Model file for the job. Use its own axes, mm. A direction names the side the tool comes from. Round coordinates to 2 decimals unless told otherwise and drop trailing zeros. Loops run counter-clockwise (first coordinate to the right, second up) from the corner with the lowest first, then second, coordinate; pieces in that order, holes last. Notation, with made-up numbers: M 66,17.5 L 86,17.5 A11 ccw 86,38.5 Z; hole C 76,87.25 d7. An arc over 180 degrees is marked long. Use a Markdown table: item, result. Add a question column.
Q1. Probe line 1 (X direction, y = 24, z = -9); line 2 (X direction, y = 4, z = 0); line 3 (Y direction, x = -8.4, z = 0). List the from-to ranges inside material, lowest first. Write a range as from..to.
Q2. Tool access for faces 5 (the face through (1.3, 3.45, -4.1)), 6 (the face through (-13, 6.9, 0)), 7 (the face through (11.13, 18.678, 0.423)), 8 (the face through (1, 3, -15)), 9 (the face through (10.8, 18, 0)): list every direction of +Z, -Z, +X, -X, +Y, -Y with a clear straight run to the whole face (end or side of a thin tool).
Q3. Mould opens along X. For faces 1 (the face through (11.62, 25.24, 0.74)), 2 (the face through (-10.8, 18, 0)), 3 (the face through (12.52, 15.3, -13.99)), 4 (the face through (-1.88, 5.2, 5.96)) say: +X half, -X half, draft (parallel to the pull), parting line (faces both ways), or undercut.
Q4. Cut at A-A (x = 0). Give the cut face in (y, z).
Q5. Cut at C-C (y = 13). Give the cut face in (x, z), plus the area to 3 significant figures.
Q6. Cut at D-D (y = 21.9). Give the cut face in (x, z), plus the area to 3 significant figures.
Q7. Pin check, flat tips, straight feed: pin 1 (6 mm diameter, centred on y = 21.9, z = 0, fed in from -X); pin 2 (10 mm diameter, centred on x = -4.5, y = 20.5, fed in from +Z); pin 3 (8.5 mm diameter, centred on y = 21.9, z = 0, fed in from +X); pin 4 (6.5 mm diameter, centred on x = 0, z = 0, fed in from +Y). Stop position of each tip, or through.
Q8. Cut at B-B (z = 0). Give the cut face in (x, y), plus the area to 3 significant figures.
from build123d import *

# Parameters (mm, degrees)
SKETCH_1_W               = 28.4
SKETCH_1_H               = 30
EXTRUDE_1_DEPTH          = 6.9
EXTRUDE_2_DEPTH          = 25
SKETCH_4_W               = 18.2
SKETCH_4_H               = 28.1
CUT_EXTRUDE_1_DEPTH      = 16
CUT_EXTRUDE_1_DEPTH_BACK = 16
CHAMFER_1_SIZE           = 2
HOLE_WIZARD_M61_D        = 5
HOLE_WIZARD_M61_DEPTH    = 3.4


with BuildPart() as part:
    # Эскиз1 → Бобышка-Вытянуть1 (new body)
    with BuildSketch(Plane(origin=(0, 0, 0), x_dir=(1, 0, 0), z_dir=(0, 1, 0))):
        Rectangle(SKETCH_1_W, SKETCH_1_H)
    extrude(amount=EXTRUDE_1_DEPTH)

    # Эскиз2 → Вырез-Повернуть1 (revolve, cut)
    with BuildSketch(Plane.XY, mode=Mode.PRIVATE) as cut_revolve_1_sk:
        Polygon((-4, 0), (-4, 3.45), (-6.25, 3.45), (-6.25, 6.9), (0, 6.9), (0, 0), align=None)
    revolve(cut_revolve_1_sk.sketch.rotate(Axis((0, 6.9, 0), (0, -1, 0)), 270), axis=Axis((0, 6.9, 0), (0, -1, 0)), mode=Mode.SUBTRACT)  # turned: the seam where the file's is

    # Эскиз3 → Бобышка-Вытянуть2 (add)
    with BuildSketch(Plane(origin=(14.2, 0, 0), x_dir=(0, 0, -1), z_dir=(1, 0, 0))):
        with BuildLine():
            Line((-15, 6.9), (-13.006126808, 23.465460141))
            ThreePointArc((-13.006126808, 23.465460141), (0, 35), (13.006126808, 23.465460141))
            Line((13.006126808, 23.465460141), (15, 6.9))
            Line((15, 6.9), (-15, 6.9))
        make_face()
    extrude(amount=-EXTRUDE_2_DEPTH)

    # Эскиз4 → Вырез-Вытянуть1 (cut, two sides)
    with BuildSketch(Plane.XY) as cut_extrude_1_sk:
        with Locations((1.7, 20.95)):
            Rectangle(SKETCH_4_W, SKETCH_4_H)
    extrude(amount=CUT_EXTRUDE_1_DEPTH, mode=Mode.SUBTRACT)
    extrude(cut_extrude_1_sk.sketch, amount=-CUT_EXTRUDE_1_DEPTH_BACK, mode=Mode.SUBTRACT)

    # Фаска1
    chamfer_1_edges = [part.edges().sort_by_distance(p)[0] for p in [
        (-14.2, 3.45, -15),
        (-14.2, 3.45, 15),
    ]]
    chamfer(chamfer_1_edges, length=CHAMFER_1_SIZE)

    # Отверстие обработанное метчиком M61
    with Locations(Plane.ZY.offset(10.8)):
        with Locations((0, 21.9)):
            Hole(HOLE_WIZARD_M61_D / 2, depth=HOLE_WIZARD_M61_DEPTH)

    # Эскиз10 → Зенковка для винта с полупотайной головкой 1 (revolve, cut)
    with BuildSketch(Plane(origin=(14.2, 21.9, 0), x_dir=(0, 0, -1), z_dir=(0, 1, 0))):
        Polygon((0, 0), (0, 3.4), (3.25, 3.4), (3.25, 2.75), (6, 0), align=None)
    revolve(axis=Axis((20.55, 21.9, 0), (-1, 0, 0)), mode=Mode.SUBTRACT)


solid = part.part
Checked values:
| question | item | result |
|---|---|---|
| 1 | line 1 | x = -10.8..-7.4, 10.8..14.2 |
| 1 | line 2 | x = -14.2..-6.25, 6.25..14.2 |
| 1 | line 3 | y = 0..19.4, 24.4..35 |
| 2 | face 5 | +Y |
| 2 | face 6 | +Z, -Z, -X, +Y |
| 2 | face 7 | +X |
| 2 | face 8 | -Z, +X, -X, +Y, -Y |
| 2 | face 9 | +Z, -Z, +Y |
| 3 | face 1 | +X half |
| 3 | face 2 | -X half |
| 3 | face 3 | draft |
| 3 | face 4 | undercut |
| 4 | outline | M 0,-15 L 6.9,-15 L 6.9,-6.25 L 3.45,-6.25 L 3.45,-4 L 0,-4 Z; M 0,4 L 3.45,4 L 3.45,6.25 L 6.9,6.25 L 6.9,15 L 0,15 Z |
| 5 | outline | M -10.8,-14.27 L -7.4,-14.27 L -7.4,14.27 L -10.8,14.27 Z; M 10.8,-14.27 L 14.2,-14.27 L 14.2,14.27 L 10.8,14.27 Z |
| 5 | area | 194 mm^2 |
| 6 | outline | M -10.8,-13.19 L -7.4,-13.19 L -7.4,-2.5 L -10.8,-2.5 Z; M -10.8,2.5 L -7.4,2.5 L -7.4,13.19 L -10.8,13.19 Z; M 10.8,-13.19 L 14.2,-13.19 L 14.2,-6 L 11.45,-3.25 L 10.8,-3.25 Z; M 10.8,3.25 L 11.45,3.25 L 14.2,6 L 14.2,13.19 L 10.8,13.19 Z |
| 6 | area | 133 mm^2 |
| 7 | pin 1 | stops at x = -10.8 |
| 7 | pin 2 | stops at z = 13.85 |
| 7 | pin 3 | stops at x = 12.45 |
| 7 | pin 4 | passes through |
| 8 | outline | M -14.2,0 L -4,0 L -4,3.45 L -6.25,3.45 L -6.25,6.9 L -7.4,6.9 L -7.4,19.4 L -10.8,19.4 L -10.8,6.9 L -14.2,6.9 Z; M -10.8,24.4 L -7.4,24.4 L -7.4,35 L -10.8,35 Z; M 4,0 L 14.2,0 L 14.2,15.9 L 11.45,18.65 L 10.8,18.65 L 10.8,6.9 L 6.25,6.9 L 6.25,3.45 L 4,3.45 Z; M 10.8,25.15 L 11.45,25.15 L 14.2,27.9 L 14.2,35 L 10.8,35 Z |
| 8 | area | 270 mm^2 |
